Check sheet for the modelled part. Datum: model origin and axes. Units: mm. Face numbers are marked on the shaded views. A direction names the side the tool comes from. Coordinates: 2 decimals unless noted, no trailing zeros. Loops run counter-clockwise (first coordinate to the right, second up) from the corner with the lowest first, then second, coordinate; pieces in that order, holes last.
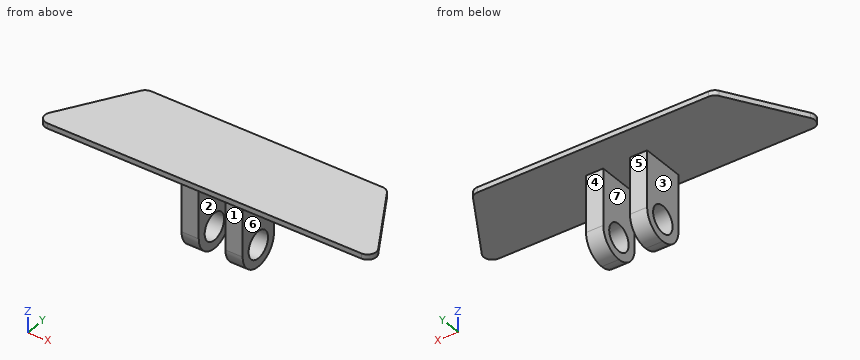
Autodesk Inventor part; units mm, degrees
ref_plane "YZ Plane" through (0, 0, 0) normal (1, 0, 0) x (0, 1, 0)
ref_plane "XZ Plane" through (0, 0, 0) normal (0, 1, 0) x (-1, 0, 0)
ref_plane "XY Plane" through (0, 0, 0) normal (0, 0, 1) x (1, 0, 0)
sketch "Sketch1" plane through (0, 0, 0) normal (0, 0, 1) x (1, 0, 0)
  line L0 (0, 31.3291) -> (70, 31.3291)
  line L1 (70, 31.3291) -> (100, -18.6709)
  line L2 (100, -18.6709) -> (0, -18.6709)
  line L3 (0, 31.3291) -> (0, -18.6709)
  line L4 (0, 31.3291) -> (-70, 31.3291)
  line L5 (-70, 31.3291) -> (-100, -18.6709)
  line L6 (-100, -18.6709) -> (0, -18.6709)
  point P0 (0, 0)
  dimension "d0" = 100
  dimension "d1" = 70
  dimension "d2" = 50
extrude "Extrusion1" add sketch "Sketch1" along normal blind 3
fillet "Fillet1" radius 5 4 edges at (70, 31.3291, 1.5) (100, -18.6709, 1.5) (-100, -18.6709, 1.5) (-70, 31.3291, 1.5)
sketch "Sketch2" plane through (0, 0, 0) normal (0, 0, -1) x (-1, 0, 0)
  line L0 (-17.75, -12.5) -> (17.75, -12.5)
  line L1 (17.75, -12.5) -> (17.75, 12.5)
  line L2 (17.75, 12.5) -> (-17.75, 12.5)
  line L3 (-17.75, 12.5) -> (-17.75, -12.5)
  line L4 (-17.75, -12.5) -> (17.75, 12.5) construction
  line L5 (17.75, -12.5) -> (-17.75, 12.5) construction
  line L6 (7.75, -12.5) -> (-7.75, -12.5)
  line L7 (-7.75, -12.5) -> (-7.75, 12.5)
  line L8 (-7.75, 12.5) -> (7.75, 12.5)
  line L9 (7.75, 12.5) -> (7.75, -12.5)
  line L10 (7.75, -12.5) -> (-7.75, 12.5) construction
  line L11 (-7.75, -12.5) -> (7.75, 12.5) construction
  point P0 (0, 0)
  dimension "d6" = 15.5
  dimension "d7" = 25
  dimension "d8" = 10
extrude "Extrusion2" add sketch "Sketch2" along normal blind 45 contours L3 L2 L7 L0 | L9 L2 L1 L0
fillet "Fillet2" radius 12.5 4 edges at (12.75, 12.5, -45) (12.75, -12.5, -45) (-12.75, -12.5, -45) (-12.75, 12.5, -45)
sketch "Sketch3" plane through (17.75, -12.5, 0) normal (1, 0, 0) x (0, 0, -1)
  arc A0 (32.5, 0) -> (32.5, 25) centre (32.5, 12.5) ccw
  line L0 (0, 25) -> (32.5, 25)
  line L1 (0, 0) -> (0, 25)
  line L2 (0, 0) -> (32.5, 0)
  circle A1 centre (32.5, 12.5) radius 7.75
  point P0 (0, 12.5)
  dimension "d12" = 15.5
extrude "Extrusion3" cut sketch "Sketch3" against normal up to surface (35.5 mm away) contours A1
properties part number "Lower Back Plate"
1) Section check D-D on x = 81. Enter the section's corners in (y, z), plus the area to 3 significant figures.
Answer sheet:
outline: (-18.67, 0) - (13, 0) - (13, 3) - (-18.67, 3) - close
area: 95.0 mm2
2) Section check B-B on y = 5. Enter the section's corners in (x, z).
Answer sheet:
outline: (-85.8, 0) - (-17.75, 0) - (-17.75, -26.58) - (-7.75, -26.58) - (-7.75, 0) - (7.75, 0) - (7.75, -26.58) - (17.75, -26.58) - (17.75, 0) - (85.8, 0) - (85.8, 3) - (-85.8, 3) - close; (-17.75, -43.96) - (-7.75, -43.96) - (-7.75, -38.42) - (-17.75, -38.42) - close; (7.75, -43.96) - (17.75, -43.96) - (17.75, -38.42) - (7.75, -38.42) - close
3) Set-up check for the marked faces 1, 2, 3 and 4: record each of +Z, -Z, +X, -X, +Y, -Y from which the full face is reachable in a straight line by a thin tool's end or side.
Answer sheet:
face 1: -Z, +X, -X, -Y
face 2: -Z, +Y, -Y
face 3: -Z, -X, +Y, -Y
face 4: -Z, +X, -X, +Y
4) Section check A-A on z = -23. Enter the section's corners in (x, y), plus the area to 3 significant figures.
Answer sheet:
outline: (-17.75, -12.5) - (-7.75, -12.5) - (-7.75, 12.5) - (-17.75, 12.5) - close; (7.75, -12.5) - (17.75, -12.5) - (17.75, 12.5) - (7.75, 12.5) - close
area: 500 mm2
5) Section check C-C on x = -50. Enter the section's corners in (y, z).
Answer sheet:
outline: (-18.67, 0) - (31.33, 0) - (31.33, 3) - (-18.67, 3) - close
6) Mould release check, pull along X, two halves, no side actions. Record for the marked faces 5, 6 and 7: +X half, -X half, draft (parallel to the pull), parting line (faces both ways), or undercut.
Answer sheet:
face 5: draft
face 6: +X half
face 7: undercut
7) Depth check by flat-ended pin: pin 1 (25 mm diameter, centred on x = -11, y = 2.5, fed in from -Z); pin 2 (20 mm diameter, centred on y = 0, z = -32.5, fed in from -X); pin 3 (3 mm diameter, centred on x = -12.5, z = -11, fed in from +Y); pin 4 (8 mm diameter, centred on x = 11, z = -10, fed in from -Y). Enter the tip coordinate at first touch or a pass-through.
Answer sheet:
pin 1: stops at z = -45
pin 2: stops at x = -17.75
pin 3: stops at y = 12.5
pin 4: stops at y = -12.5
8) Scan lines: line 1 (X direction, y = 8, z = -22.5); line 2 (Y direction, x = 11.75, z = -32.5); line 3 (Z direction, x = 78.5, y = 1). Record each from-to range of solid material in increasing order.
Answer sheet:
line 1: x = -17.75 to -7.75, 7.75 to 17.75
line 2: y = -12.5 to -7.75, 7.75 to 12.5
line 3: z = 0 to 3
